from build123d import *

# Parameters (mm, degrees)
F1_DEPTH = 20
F2_R     = 2.5
F3_DEPTH = 2.001
F4_R     = 2.5
F5_DEPTH = 25


with BuildPart() as f1:
    # F0 (on Front) → F1 (new body, symmetric)
    with BuildSketch(Plane.XZ):
        with BuildLine():
            Line((-92.5, 2), (-92.5, 0))
            Line((-92.5, 0), (-78, 0))
            ThreePointArc((-78, 0), (-75.171573, 1.171573), (-74, 4))
            Line((-74, 4), (-74, 66))
            ThreePointArc((-74, 66), (-73.414214, 67.414214), (-72, 68))
            Line((-72, 68), (0, 68))
            Line((0, 68), (72, 68))
            ThreePointArc((72, 68), (73.414214, 67.414214), (74, 66))
            Line((74, 66), (74, 4))
            ThreePointArc((74, 4), (75.171573, 1.171573), (78, 0))
            Line((78, 0), (92.5, 0))
            Line((92.5, 0), (92.5, 2))
            Line((92.5, 2), (78, 2))
            ThreePointArc((78, 2), (76.585786, 2.585786), (76, 4))
            Line((76, 4), (76, 66))
            ThreePointArc((76, 66), (74.828427, 68.828427), (72, 70))
            Line((72, 70), (0, 70))
            Line((0, 70), (-72, 70))
            ThreePointArc((-72, 70), (-74.828427, 68.828427), (-76, 66))
            Line((-76, 66), (-76, 4))
            ThreePointArc((-76, 4), (-76.585786, 2.585786), (-78, 2))
            Line((-78, 2), (-92.5, 2))
        make_face()
    extrude(amount=F1_DEPTH, both=True)

    # F2 (on face) → F3 (cut, through all)
    with BuildSketch(Plane.XY.offset(2)):
        with Locations((-85, 0)):
            Circle(F2_R)
        with Locations((85, 0)):
            Circle(F2_R)
    extrude(amount=-F3_DEPTH, mode=Mode.SUBTRACT)

    # F4 (on face) → F5 (cut)
    with BuildSketch(Plane.XY.offset(70)):
        with Locations((-30, 0)):
            Circle(F4_R)
        with Locations((30, 0)):
            Circle(F4_R)
    extrude(amount=-F5_DEPTH, mode=Mode.SUBTRACT)


solid = f1.part
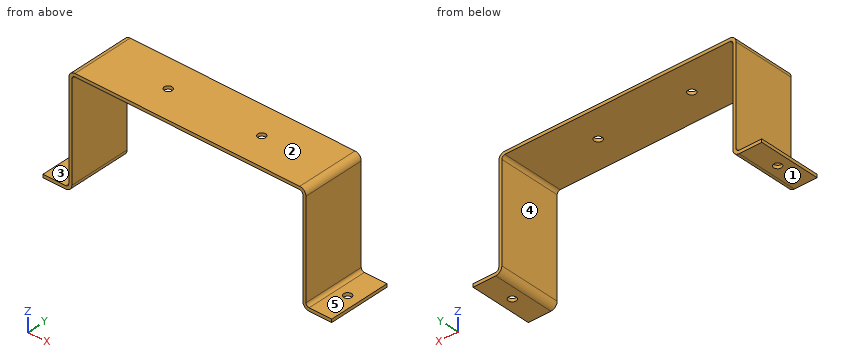
Build history of the part. All positions in model axes, mm. Face numbers are marked on the shaded views. A direction names the side the tool comes from. Coordinates: 2 decimals unless noted, no trailing zeros. Write each loop counter-clockwise with the first axis right and the second up, starting at its lowest first coordinate (ties: lowest second). Pieces come first, ordered by that corner, then holes.
(1) Cut at B-B on z = 52.5. List the corners of the cut face in (x, y).
(2) Drill centre lines: line 1 (X direction, y = 14, z = 14.5); line 2 (Z direction, x = -36.5, y = 14); line 3 (X direction, y = -4, z = 66.5). Where is each one in solid material? Low to high.
(3) Cut at A-A on x = -85. List the corners of the cut face in (y, z).
(4) Pin check, flat tips, straight feed: pin 1 Ø12 at (y, z) = (-6, 40) entering from -X; pin 2 Ø8 at (y, z) = (6, 33) entering from +X; pin 3 Ø12 at (x, y) = (15, -12.5) entering from -Z. Stop position of each tip, or through.
(5) Cut at C-C on y = 16. List the corners of the cut face in (x, z).
(6) Cut at D-D on y = 0. State how many separate pieces and enclosed holes the cut face has, and give its area (3 significant figures).
(7) 3-axis set-ups, long thin cutter, end or side, ignore diameter. For the marked faces 1, 2, 3, 4 and 5: which of +Z, -Z, +X, -X, +Y, -Y reach the whole face in a straight line?
Working result:
1. outline: (-76, -20) - (-74, -20) - (-74, 20) - (-76, 20) - close; (74, -20) - (76, -20) - (76, 20) - (74, 20) - close
2. line 1: x = -76 to -74, 74 to 76
2. line 2: z = 68 to 70
2. line 3: x = -75.97 to -73.94, 73.94 to 75.97
3. outline: (-20, 0) - (-2.5, 0) - (-2.5, 2) - (-20, 2) - close; (2.5, 0) - (20, 0) - (20, 2) - (2.5, 2) - close
4. pin 1: stops at x = -76
4. pin 2: stops at x = 76
4. pin 3: stops at z = 68
5. outline: (-92.5, 0) - (-78, 0) arc R4 ccw to (-74, 4) - (-74, 66) arc R2 cw to (-72, 68) - (72, 68) arc R2 cw to (74, 66) - (74, 4) arc R4 ccw to (78, 0) - (92.5, 0) - (92.5, 2) - (78, 2) arc R2 cw to (76, 4) - (76, 66) arc R4 ccw to (72, 70) - (-72, 70) arc R4 ccw to (-76, 66) - (-76, 4) arc R2 cw to (-78, 2) - (-92.5, 2) - close
6. separate pieces: 5
6. enclosed holes: 0
6. area: 592 mm2
7. face 1: -Z, +X, -X, +Y, -Y
7. face 2: +Z, +X, -X, +Y, -Y
7. face 3: +Z, -X, +Y, -Y
7. face 4: -Z, +Y, -Y
7. face 5: +Z, +X, +Y, -Y
